```python
from build123d import *

# Parameters (mm, degrees)
ESBO_O1_R                = 14
ESBO_O1_R_2              = 11.25
RESSALTO_EXTRUS_O1_DEPTH = 3.5
ESBO_O2_W                = 60
ESBO_O2_H                = 4
RESSALTO_EXTRUS_O2_DEPTH = 6
CHANFRO3_SIZE            = 10
CHANFRO5_SIZE            = 10
ESBO_O6_R                = 2.1
CORTE_EXTRUS_O2_DEPTH    = 51.89449872
ESBO_O7_R                = 4.9
CORTE_EXTRUS_O6_DEPTH    = 51.89449872
FILETE1_R                = 3


with BuildPart() as part:
    # Esboço1 → Ressalto-extrusão1 (new, symmetric)
    # profile 1 of 3: a face of its own
    with BuildSketch(Plane(origin=(0, 0, 0), x_dir=(1, 0, 0), z_dir=(0, 1, 0))):
        Polygon((30, 22), (-30, 22), (-30, 18), (-14, 18), (14, 18), (30, 18), align=None)
    # profile 2 of 3: a face of its own
    with BuildSketch(Plane(origin=(0, 0, 0), x_dir=(1, 0, 0), z_dir=(0, 1, 0))):
        with BuildLine():
            Line((14, 18), (-14, 18))
            Line((-14, 18), (-14, -8))
            ThreePointArc((-14, -8), (0, 6), (14, -8))
            Line((14, -8), (14, 18))
        make_face()
    # profile 3 of 3: a face of its own
    with BuildSketch(Plane(origin=(0, 0, 0), x_dir=(1, 0, 0), z_dir=(0, 1, 0))):
        with Locations((0, -8)):
            Circle(ESBO_O1_R)
        with Locations(Location((0, -8, 0), (0, 0, 270))):
            Circle(ESBO_O1_R_2, mode=Mode.SUBTRACT)
    extrude(amount=RESSALTO_EXTRUS_O1_DEPTH, both=True)

    # Esboço2 → Ressalto-extrusão2 (add)
    with BuildSketch(Plane(origin=(0, 3.5, 0), x_dir=(1, 0, 0), z_dir=(0, 1, 0))):
        with Locations((0, 20)):
            Rectangle(ESBO_O2_W, ESBO_O2_H)
    extrude(amount=RESSALTO_EXTRUS_O2_DEPTH)

    # Chanfro3
    chanfro3_edges = [part.edges().sort_by_distance(p)[0] for p in [
        (14, 0, -18),
        (-14, 0, -18),
    ]]
    chamfer(chanfro3_edges, length=CHANFRO3_SIZE)

    # Chanfro5
    # the kernel refuses this chamfer: 10 mm, written as the material it adds along each edge
    with BuildSketch(Plane(origin=(-49.71682988, 3.5, -18), x_dir=(0, 0.9996219169112968, -0.027495876610586317), z_dir=(1, 0, 0))) as chanfro5_piece_1_section:
        Polygon((CHANFRO5_SIZE * 0.999621916911, CHANFRO5_SIZE * 0.0274958766106), (-CHANFRO5_SIZE * 0.0274958766106, CHANFRO5_SIZE * 0.999621916911), (0, 0), align=None)
    chanfro5_piece_1 = extrude(amount=99.433659759, mode=Mode.PRIVATE)
    chanfro5_piece_1 = split(chanfro5_piece_1, bisect_by=Plane(origin=(-17.624703453, 9.5, -15.249406907), z_dir=(0, -1, 0)), keep=Keep.TOP, mode=Mode.PRIVATE)
    chanfro5_piece_1 = split(chanfro5_piece_1, bisect_by=Plane(origin=(-19.43705518, 6.203831668, -13.43705518), z_dir=(0.7071067811865475, 0, -0.7071067811865477)), keep=Keep.TOP, mode=Mode.PRIVATE)
    chanfro5_piece_1 = split(chanfro5_piece_1, bisect_by=Plane(origin=(-14, 6.203831668, -15.249406907), z_dir=(-1, 0, 0)), keep=Keep.TOP, mode=Mode.PRIVATE)
    add(chanfro5_piece_1)
    with BuildSketch(Plane(origin=(-49.71682988, 3.5, -18), x_dir=(0, 0.9996219169112968, -0.027495876610586317), z_dir=(1, 0, 0))) as chanfro5_piece_2_section:
        Polygon((CHANFRO5_SIZE * 0.999621916911, CHANFRO5_SIZE * 0.0274958766106), (-CHANFRO5_SIZE * 0.0274958766106, CHANFRO5_SIZE * 0.999621916911), (0, 0), align=None)
    chanfro5_piece_2 = extrude(amount=99.433659759, mode=Mode.PRIVATE)
    chanfro5_piece_2 = split(chanfro5_piece_2, bisect_by=Plane(origin=(0, 9.5, -14.250020725), z_dir=(0, -1, 0)), keep=Keep.TOP, mode=Mode.PRIVATE)
    chanfro5_piece_2 = split(chanfro5_piece_2, bisect_by=Plane(origin=(10.125010362, 5.933615653, -4.125010362), z_dir=(-0.7071067811865479, 0, -0.7071067811865474)), keep=Keep.TOP, mode=Mode.PRIVATE)
    chanfro5_piece_2 = split(chanfro5_piece_2, bisect_by=Plane(origin=(14, 5.933615653, -14.250020725), z_dir=(-1, 0, 0)), keep=Keep.TOP, mode=Mode.PRIVATE)
    chanfro5_piece_2 = split(chanfro5_piece_2, bisect_by=Plane(origin=(-14, 5.933615653, -14.250020725), z_dir=(1, 0, 0)), keep=Keep.TOP, mode=Mode.PRIVATE)
    add(chanfro5_piece_2)
    with BuildSketch(Plane(origin=(-49.71682988, 3.5, -18), x_dir=(0, 0.9996219169112968, -0.027495876610586317), z_dir=(1, 0, 0))) as chanfro5_piece_3_section:
        Polygon((CHANFRO5_SIZE * 0.999621916911, CHANFRO5_SIZE * 0.0274958766106), (-CHANFRO5_SIZE * 0.0274958766106, CHANFRO5_SIZE * 0.999621916911), (0, 0), align=None)
    chanfro5_piece_3 = extrude(amount=99.433659759, mode=Mode.PRIVATE)
    chanfro5_piece_3 = split(chanfro5_piece_3, bisect_by=Plane(origin=(17.624703453, 9.5, -15.249406907), z_dir=(0, -1, 0)), keep=Keep.TOP, mode=Mode.PRIVATE)
    chanfro5_piece_3 = split(chanfro5_piece_3, bisect_by=Plane(origin=(19.43705518, 6.203831668, -13.43705518), z_dir=(-0.7071067811865479, 0, -0.7071067811865474)), keep=Keep.TOP, mode=Mode.PRIVATE)
    chanfro5_piece_3 = split(chanfro5_piece_3, bisect_by=Plane(origin=(14, 6.203831668, -15.249406907), z_dir=(1, 0, 0)), keep=Keep.TOP, mode=Mode.PRIVATE)
    add(chanfro5_piece_3)

    # Esboço6 → Corte-extrusão2 (cut, symmetric)
    with BuildSketch(Plane.XY.offset(-18)):
        with Locations((-25, 3)):
            Circle(ESBO_O6_R)
    corte_extrus_o2 = extrude(amount=CORTE_EXTRUS_O2_DEPTH, both=True, mode=Mode.SUBTRACT)

    # Esboço7 → Corte-extrusão6 (cut, through all)
    with BuildSketch(Plane.XY.offset(-18)):
        with Locations((-25, 3)):
            Circle(ESBO_O7_R)
    corte_extrus_o6 = extrude(amount=CORTE_EXTRUS_O6_DEPTH, mode=Mode.SUBTRACT)

    # Espelhar2: Corte-extrusão2, Corte-extrusão6 across plane
    add(corte_extrus_o2.mirror(Plane(origin=(0, 0, 0), x_dir=(0, 0, 1), z_dir=(1, 0, 0))), mode=Mode.SUBTRACT)
    add(corte_extrus_o6.mirror(Plane(origin=(0, 0, 0), x_dir=(0, 0, 1), z_dir=(1, 0, 0))), mode=Mode.SUBTRACT)

    # Filete1
    filete1_edges = [part.edges().sort_by_distance(p)[0] for p in [
        (30, -3.5, -20),
        (-30, -3.5, -20),
        (-30, 9.5, -20),
        (30, 9.5, -20),
    ]]
    fillet(filete1_edges, radius=FILETE1_R)


solid = part.part
```
Can you work these out from the model? Positions are in its coordinate system, mm. A direction names the side the tool comes from. Coordinates: 2 decimals unless noted, no trailing zeros. Order: outer loops, then holes, each group sorted by start corner. A loop starts at its lowest first (then second) coordinate and runs counter-clockwise, first axis right, second up. Notation, with made-up numbers: (-37, 47.25) - (-3, 47.25) arc R20 cw to (-3, 81.25) - close; hole circle Ø6 at (58.25, 45). An arc over 180 degrees is marked (long way). Answer in a Markdown table with one row per item.
1. Suppose I cut it at C-C (z = 3.5). Please give me the cut outline in (x, y).
Reply:
| item | result |
|---|---|
| outline | (-14, -3.5) - (-10.31, -3.5) - (-10.31, 3.5) - (-14, 3.5) - close; (10.31, -3.5) - (14, -3.5) - (14, 3.5) - (10.31, 3.5) - close |
2. For pin 1 (2 mm diameter, centred on y = 1, z = 0, fed in from +X); pin 2 (4 mm diameter, centred on y = 1, z = -7.5, fed in from -X); pin 3 (5 mm diameter, centred on x = 27.5, y = 3.5, fed in from +Z), each with a flat end and sliding along its axis, tell me the tip position at first contact or that it passes through.
Reply:
| item | result |
|---|---|
| pin 1 | stops at x = 14 |
| pin 2 | stops at x = -15.5 |
| pin 3 | stops at z = -18 |
3. Suppose I cut it at D-D (x = 0). Please give me the cut outline in (y, z).
Reply:
| item | result |
|---|---|
| outline | (-3.5, -22) - (9.5, -22) - (9.5, -14) - (3.5, -8) - (3.5, -3.25) - (-3.5, -3.25) - close; (-3.5, 19.25) - (3.5, 19.25) - (3.5, 22) - (-3.5, 22) - close |
4. If we mould it in two halves opening along Y, with no side actions, what happens to faces 1 (the cylindrical face through (-29.1, -2.64, -19.97)), 2 (the flat face through (27.2, 4.4, -18)), 3 (the flat face through (14, 0, 0)), 4 (the cylindrical face through (-29.1, 8.64, -20.03))? For each: pulls with the +Y half, pulls with the -Y half, needs draft (parallel to the pull), parting line crosses it, or undercut.
Reply:
| item | result |
|---|---|
| face 1 | pulls with the -Y half |
| face 2 | undercut |
| face 3 | needs draft |
| face 4 | pulls with the +Y half |
5. Suppose I cut it at A-A (x = -25). Please give me the cut outline in (y, z).
Reply:
| item | result |
|---|---|
| outline | (-3.5, -22) - (0.9, -22) - (0.9, -18) - (-3.5, -18) - close; (5.1, -22) - (9.5, -22) - (9.5, -18) - (5.1, -18) - close |
6. If I drill on line 1 along Y through (x, z) = (-25, -20.5); line 2 along X through (y, z) = (1.5, -19); line 3 along X through (y, z) = (-3, 7.5), over which ranges is the centre line in solid material (lowest first)?
Reply:
| item | result |
|---|---|
| line 1 | y = -3.5 to 0.9, 5.1 to 9.5 |
| line 2 | x = -30 to -26.47, -23.53 to 23.53, 26.47 to 30 |
| line 3 | x = -14 to -11.24, 11.24 to 14 |
7. Suppose I cut it at B-B (y = 4.25). Please give me the cut outline in (x, z).
Reply:
| item | result |
|---|---|
| outline | (-30, -22) - (-26.69, -22) - (-26.69, -18) - (-30, -18) - close; (-23.31, -22) - (23.31, -22) - (23.31, -18) - (20.26, -18) - (20.26, -14.26) - (14.75, -8.75) - (-14.75, -8.75) - (-20.26, -14.26) - (-20.26, -18) - (-23.31, -18) - close; (26.69, -22) - (30, -22) - (30, -18) - (26.69, -18) - close |
8. For faces 5 (the flat face through (-27.3, 2.9, -18)), 6 (the flat face through (19, 1, -13)), 7 (the cylindrical face through (29.1, 8.64, -20.03)), 8 (the flat face through (3, 3.5, -3)), 9 (the flat face through (-14, 0, 0)), which set-ups out of +Z, -Z, +X, -X, +Y, -Y let a thin tool reach every point of the face, with its end or its side?
Reply:
| item | result |
|---|---|
| face 5 | +Z, -X |
| face 6 | +Z, +X, +Y, -Y |
| face 7 | +Z, -Z, +X, +Y |
| face 8 | +Z, +X, -X, +Y |
| face 9 | +Z, -X, +Y, -Y |
